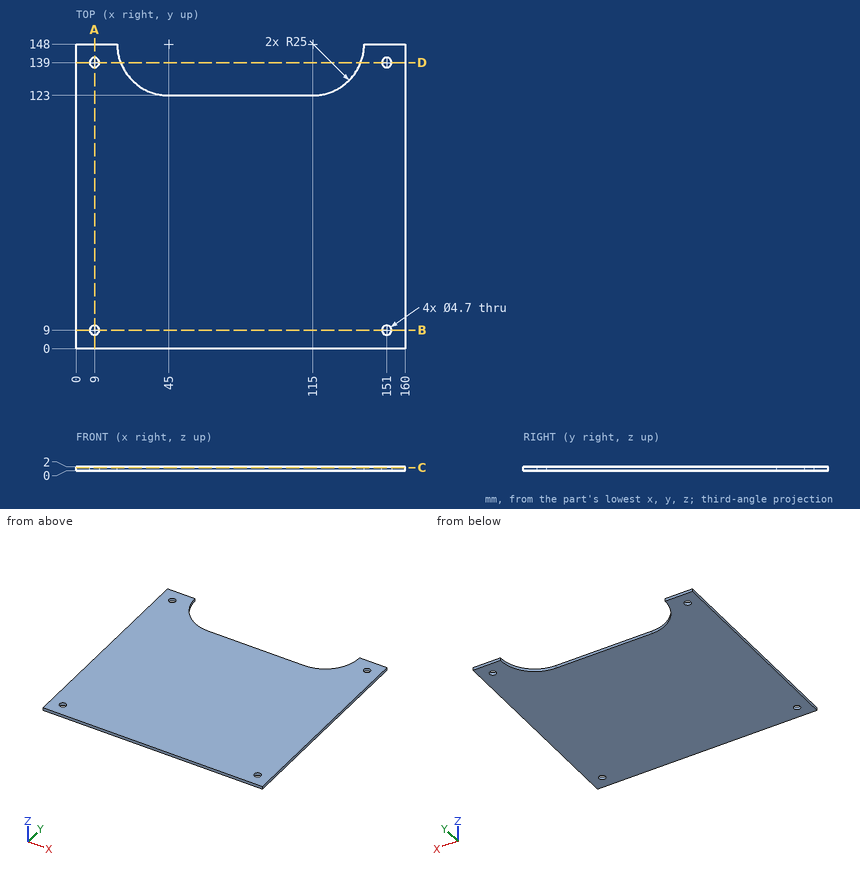
Design review of the part shown in the three views and the two pictorial views. Dimensions are in mm from the part's minimum x, y and z. Coordinates: 2 decimals unless noted, no trailing zeros. Order: outer loops, then holes, each group sorted by start corner. A loop starts at its lowest first (then second) coordinate and runs counter-clockwise, first axis right, second up.
Item 1: Take a section at B-B, the plane y = 9. Write out the cut boundary in (x, z).
Item 2: Take a section at C-C, the plane z = 1.55. Write out the cut boundary in (x, y).
Item 3: For pin 1 Ø4 at (x, y) = (151, 9) entering from -Z, flat-tipped, find the tip position at first contact; note if it passes through.
Item 4: Take a section at D-D, the plane y = 139. Write out the cut boundary in (x, z), then the cut area to 3 significant figures.
Item 5: Take a section at A-A, the plane x = 9. Write out the cut boundary in (y, z).
Item 6: For line 1 (Y direction, x = 151, z = 0.6); line 2 (X direction, y = 139, z = 0.5); line 3 (Y direction, x = 53.5, z = 1.15), list the stretches that pass through material, from the lowest coordinate up.
The answers:
1. outline: (0, 0) - (6.65, 0) - (6.65, 2) - (0, 2) - close; (11.35, 0) - (148.65, 0) - (148.65, 2) - (11.35, 2) - close; (153.35, 0) - (160, 0) - (160, 2) - (153.35, 2) - close
2. outline: (0, 0) - (160, 0) - (160, 148) - (140, 148) arc R25 cw to (115, 123) - (45, 123) arc R25 cw to (20, 148) - (0, 148) - close; hole circle Ø4.7 at (9, 9); hole circle Ø4.7 at (9, 139); hole circle Ø4.7 at (151, 9); hole circle Ø4.7 at (151, 139)
3. pin 1: passes through
4. outline: (0, 0) - (6.65, 0) - (6.65, 2) - (0, 2) - close; (11.35, 0) - (21.68, 0) - (21.68, 2) - (11.35, 2) - close; (138.32, 0) - (148.65, 0) - (148.65, 2) - (138.32, 2) - close; (153.35, 0) - (160, 0) - (160, 2) - (153.35, 2) - close
4. area: 67.9 mm2
5. outline: (0, 0) - (6.65, 0) - (6.65, 2) - (0, 2) - close; (11.35, 0) - (136.65, 0) - (136.65, 2) - (11.35, 2) - close; (141.35, 0) - (148, 0) - (148, 2) - (141.35, 2) - close
6. line 1: y = 0 to 6.65, 11.35 to 136.65, 141.35 to 148
6. line 2: x = 0 to 6.65, 11.35 to 21.68, 138.32 to 148.65, 153.35 to 160
6. line 3: y = 0 to 123
